```python
from build123d import *

# Parameters (mm, degrees)
SKETCH1_W                = 12.7
SKETCH1_H                = 271.365530146
BOSS_EXTRUDE1_DEPTH      = 248.25
SKETCH2_W                = 172.05
SKETCH2_H                = 118.965530146
CUT_EXTRUDE1_DEPTH       = 312.978479114
FILLET1_R                = 50.8
HOLE1_D                  = 3.175
HOLE1_DEPTH              = 31.75
HOLE1_CSINK_D            = 10.16
HOLE1_CSINK_ANGLE        = 82
HOLE1_TIP                = 0.953866233
HOLE2_D                  = 3.175
HOLE2_DEPTH              = 31.75
HOLE2_CSINK_D            = 10.16
HOLE2_CSINK_ANGLE        = 82
HOLE2_TIP                = 0.953866233
F_5_16_CLEARANCE_HOLE1_D = 8.72998


with BuildPart() as part:
    # Sketch1 → Boss-Extrude1 (new body)
    with BuildSketch(Plane.XY):
        with Locations((-228.402967181, -52.841023691)):
            Rectangle(SKETCH1_W, SKETCH1_H)
    extrude(amount=BOSS_EXTRUDE1_DEPTH)

    # Sketch2 → Cut-Extrude1 (cut, through all)
    with BuildSketch(Plane.ZY.offset(234.752967181)):
        with Locations((124.125, -52.841023691)):
            Rectangle(SKETCH2_W, SKETCH2_H)
    extrude(amount=-CUT_EXTRUDE1_DEPTH, mode=Mode.SUBTRACT)

    # Fillet1
    fillet1_edges = [part.edges().sort_by_distance(p)[0] for p in [
        (-228.402967181, 6.641741382, 210.15),
        (-228.402967181, -112.323788764, 210.15),
        (-228.402967181, -112.323788764, 38.1),
        (-228.402967181, 6.641741382, 38.1),
    ]]
    fillet(fillet1_edges, radius=FILLET1_R)

    # Hole1
    with Locations(Plane(origin=(181.039434513, -52.974999997, -12.7), x_dir=(0, -1, 0), z_dir=(0, 0, -1))):
        with Locations((129.198788767, 384.042401694), (-129.466741379, 384.042401694), (-129.466741379, 304.786761906), (-110.416741379, 409.442401694), (-0.133976306, 409.442401694), (110.148788767, 409.442401694), (129.198788767, 304.786761906)):
            CounterSinkHole(HOLE1_D / 2, HOLE1_CSINK_D / 2, depth=HOLE1_DEPTH, counter_sink_angle=HOLE1_CSINK_ANGLE)
            with Locations((0, 0, -(HOLE1_DEPTH + HOLE1_TIP / 2))):  # 118° drill point
                Cone(0, HOLE1_D / 2, HOLE1_TIP, mode=Mode.SUBTRACT)

    # Hole2
    with Locations(Plane(origin=(-234.752967181, -52.974999997, -1073.364195846), x_dir=(0, -1, 0), z_dir=(-1, 0, 0))):
        with Locations((-129.466741379, 1300.662770337), (-129.466741379, 1128.612770337), (129.198788767, 1128.612770337), (129.198788767, 1300.662770337)):
            CounterSinkHole(HOLE2_D / 2, HOLE2_CSINK_D / 2, depth=HOLE2_DEPTH, counter_sink_angle=HOLE2_CSINK_ANGLE)
            with Locations((0, 0, -(HOLE2_DEPTH + HOLE2_TIP / 2))):  # 118° drill point
                Cone(0, HOLE2_D / 2, HOLE2_TIP, mode=Mode.SUBTRACT)

    # 5/16 Clearance Hole1 (through all)
    with Locations(Plane.ZY.offset(234.752967181)):
        with Locations((206.1876, -167.467547412), (206.1876, 61.78550003), (29.3624, 61.78550003), (29.3624, -167.467547412)):
            Hole(F_5_16_CLEARANCE_HOLE1_D / 2)


solid = part.part
```
Model file for the job. Use its own axes, mm. A direction names the side the tool comes from. Give positions to 0.01 mm unless a question says otherwise; leave off trailing zeros. Write each loop counter-clockwise with the first axis right and the second up, starting at its lowest first coordinate (ties: lowest second). Pieces come first, ordered by that corner, then holes. Notation, with made-up numbers: (39, 3) - (89, 3) arc R16 cw to (89, 30) - close; hole circle Ø3 at (38, -31.5). An arc over 180 degrees is marked (long way). One line per question, with ' | ' between items. Start each with the question number.
(1) 3-axis set-ups, long thin cutter, end or side, ignore diameter. For faces 4 (the face through (-228, -53, 210.15)), 5 (the face through (-234.753, -115, 122)): which of +Z, -Z, +X, -X, +Y, -Y reach the whole face in a straight line?
(2) Wall check: line 1 along Z through (x, y) = (-222.75, -43); line 2 along Y through (x, z) = (-227, 141); line 3 along Z through (x, y) = (-227.5, -55.5). Give the ranges that are in metal, low to high. Write a range as from..to.
(3) Two-plate mould, pull along Y, no slides. Class faces 1 (the face through (-228, -51, 0)), 2 (the face through (-228, -188.524, 122)), 3 (the face through (-230.93, 77.3, 53.69)): +Y half, -Y half, draft (parallel to the pull), parting line (faces both ways), or undercut.
(4) Pin check, flat tip, straight feed: P1, Ø4, axis at y = 76.49, z = 227.3, coming from the -X side. Stop position of the tip, or through.
(5) Slice it at B-B on y = 0. Write the cut outline in (x, z), plus the area to 3 significant figures.
(6) Slice it at A-A on z = 119. Write the cut outline in (x, y), plus the area to 3 significant figures.
(7) Slice it at C-C on x = -232.75. Give the number of separate pieces and of enclosed holes in the cut face, plus the area to 3 significant figures.
Results below:
1) face 4: +X, -X | face 5: +Z, -Z, -X, +Y, -Y
2) line 1: 0..38.11, 210.14..248.25 | line 2: -188.52..-112.32, 6.64..82.84 | line 3: 0..38.1, 210.15..248.25
3) face 1: draft | face 2: -Y half | face 3: undercut
4) P1: x = -231.21
5) outline: (-234.75, 0) - (-222.05, 0) - (-222.05, 63.79) - (-234.75, 63.79) - close; (-234.75, 184.46) - (-222.05, 184.46) - (-222.05, 248.25) - (-234.75, 248.25) - close | area: 1,620 mm^2
6) outline: (-234.75, -188.52) - (-222.05, -188.52) - (-222.05, -112.32) - (-234.75, -112.32) - close; (-234.75, 6.64) - (-222.05, 6.64) - (-222.05, 82.84) - (-234.75, 82.84) - close | area: 1,940 mm^2
7) separate pieces: 1 | enclosed holes: 9 | area: 48,700 mm^2
